Geometry: final body of the model. Coordinates: model frame, mm. Give positions to 0.01 mm unless a question says otherwise; leave off trailing zeros. Write each loop counter-clockwise with the first axis right and the second up, starting at its lowest first coordinate (ties: lowest second). Pieces come first, ordered by that corner, then holes.
```python
from build123d import *

# Parameters (mm, degrees)
F0_R     = 1.75
F1_DEPTH = 2.5


with BuildPart() as f1:
    # F0 (on Top) → F1 (new body)
    with BuildSketch(Plane.XY):
        with BuildLine():
            ThreePointArc((-38.5, -35.5), (-37.62132, -37.62132), (-35.5, -38.5))
            Line((-35.5, -38.5), (-2, -38.5))
            Line((-2, -38.5), (-2, -38.448017))
            ThreePointArc((-2, -38.448017), (-1.000338, -38.487002), (0, -38.5))
            ThreePointArc((0, -38.5), (1.000338, -38.487002), (2, -38.448017))
            Line((2, -38.448017), (2, -38.5))
            Line((2, -38.5), (35.5, -38.5))
            ThreePointArc((35.5, -38.5), (37.62132, -37.62132), (38.5, -35.5))
            Line((38.5, -35.5), (38.5, -2))
            Line((38.5, -2), (38.448017, -2))
            ThreePointArc((38.448017, -2), (38.487002, -1.000338), (38.5, 0))
            ThreePointArc((38.5, 0), (38.487002, 1.000338), (38.448017, 2))
            Line((38.448017, 2), (38.5, 2))
            Line((38.5, 2), (38.5, 35.5))
            ThreePointArc((38.5, 35.5), (37.62132, 37.62132), (35.5, 38.5))
            Line((35.5, 38.5), (2, 38.5))
            Line((2, 38.5), (2, 38.448017))
            ThreePointArc((2, 38.448017), (1.000338, 38.487002), (0, 38.5))
            ThreePointArc((0, 38.5), (-1.000338, 38.487002), (-2, 38.448017))
            Line((-2, 38.448017), (-2, 38.5))
            Line((-2, 38.5), (-35.5, 38.5))
            ThreePointArc((-35.5, 38.5), (-37.62132, 37.62132), (-38.5, 35.5))
            Line((-38.5, 35.5), (-38.5, 2))
            Line((-38.5, 2), (-38.448017, 2))
            ThreePointArc((-38.448017, 2), (-38.487002, 1.000338), (-38.5, 0))
            ThreePointArc((-38.5, 0), (-38.487002, -1.000338), (-38.448017, -2))
            Line((-38.448017, -2), (-38.5, -2))
            Line((-38.5, -2), (-38.5, -35.5))
        make_face()
        with Locations((-35, -35)):
            Circle(F0_R, mode=Mode.SUBTRACT)
        with BuildLine():
            Line((-16.039015, -35), (-31.045212, -35))
            ThreePointArc((-31.045212, -35), (-31.075605, -34.510637), (-31.166319, -34.028796))
            Line((-31.166319, -34.028796), (-25.754724, -28.617201))
            ThreePointArc((-25.754724, -28.617201), (-21.139162, -32.177412), (-16.039015, -35))
        make_face(mode=Mode.SUBTRACT)
        with BuildLine():
            ThreePointArc((-33.974785, -31.180408), (-34.482954, -31.079157), (-35, -31.045212))
            Line((-35, -31.045212), (-35, -16.039015))
            ThreePointArc((-35, -16.039015), (-32.164167, -21.159309), (-28.584922, -25.790545))
            Line((-28.584922, -25.790545), (-33.974785, -31.180408))
        make_face(mode=Mode.SUBTRACT)
        with BuildLine():
            Line((-2, -28.429738), (-2, -34.94281))
            ThreePointArc((-2, -34.94281), (-24.748737, -24.748737), (-34.94281, -2))
            Line((-34.94281, -2), (-28.429738, -2))
            ThreePointArc((-28.429738, -2), (-20.152543, -20.152543), (-2, -28.429738))
        make_face(mode=Mode.SUBTRACT)
        with BuildLine():
            Line((-2, -4.862478), (-2, -14.866069))
            ThreePointArc((-2, -14.866069), (-10.606602, -10.606602), (-14.866069, -2))
            Line((-14.866069, -2), (-4.794377, -2))
            Line((-4.794377, -2), (-8.49896, -8.49896))
            Line((-8.49896, -8.49896), (-2, -4.862478))
        make_face(mode=Mode.SUBTRACT)
        with BuildLine():
            ThreePointArc((-11.571705, -14.434183), (0.024219, -18.499984), (11.609459, -14.403835))
            Line((11.609459, -14.403835), (16.22518, -19.019557))
            ThreePointArc((16.22518, -19.019557), (0.024155, -24.999988), (-16.188397, -19.050874))
            Line((-16.188397, -19.050874), (-11.571705, -14.434183))
        make_face(mode=Mode.SUBTRACT)
        with BuildLine():
            Line((25.790545, -28.584922), (31.180408, -33.974785))
            ThreePointArc((31.180408, -33.974785), (31.079157, -34.482954), (31.045212, -35))
            Line((31.045212, -35), (16.039015, -35))
            ThreePointArc((16.039015, -35), (21.159309, -32.164167), (25.790545, -28.584922))
        make_face(mode=Mode.SUBTRACT)
        with Locations((35, -35)):
            Circle(F0_R, mode=Mode.SUBTRACT)
        with BuildLine():
            Line((35, -16.039015), (35, -31.045212))
            ThreePointArc((35, -31.045212), (34.510637, -31.075605), (34.028796, -31.166319))
            Line((34.028796, -31.166319), (28.617201, -25.754724))
            ThreePointArc((28.617201, -25.754724), (32.177412, -21.139162), (35, -16.039015))
        make_face(mode=Mode.SUBTRACT)
        with BuildLine():
            ThreePointArc((2, -28.429738), (20.152543, -20.152543), (28.429738, -2))
            Line((28.429738, -2), (34.94281, -2))
            ThreePointArc((34.94281, -2), (24.748737, -24.748737), (2, -34.94281))
            Line((2, -34.94281), (2, -28.429738))
        make_face(mode=Mode.SUBTRACT)
        with BuildLine():
            ThreePointArc((14.866069, -2), (10.606602, -10.606602), (2, -14.866069))
            Line((2, -14.866069), (2, -4.862478))
            Line((2, -4.862478), (8.49896, -8.49896))
            Line((8.49896, -8.49896), (4.794377, -2))
            Line((4.794377, -2), (14.866069, -2))
        make_face(mode=Mode.SUBTRACT)
        with BuildLine():
            ThreePointArc((-19.019557, -16.22518), (-25, 0), (-19.019557, 16.22518))
            Line((-19.019557, 16.22518), (-14.403835, 11.609459))
            ThreePointArc((-14.403835, 11.609459), (-18.5, 0), (-14.403835, -11.609459))
            Line((-14.403835, -11.609459), (-19.019557, -16.22518))
        make_face(mode=Mode.SUBTRACT)
        with BuildLine():
            ThreePointArc((-14.866069, 2), (-10.606602, 10.606602), (-2, 14.866069))
            Line((-2, 14.866069), (-2, 4.862478))
            Line((-2, 4.862478), (-8.49896, 8.49896))
            Line((-8.49896, 8.49896), (-4.794377, 2))
            Line((-4.794377, 2), (-14.866069, 2))
        make_face(mode=Mode.SUBTRACT)
        with BuildLine():
            ThreePointArc((-34.94281, 2), (-24.748737, 24.748737), (-2, 34.94281))
            Line((-2, 34.94281), (-2, 28.429738))
            ThreePointArc((-2, 28.429738), (-20.152543, 20.152543), (-28.429738, 2))
            Line((-28.429738, 2), (-34.94281, 2))
        make_face(mode=Mode.SUBTRACT)
        with BuildLine():
            Line((-33.974785, 31.180408), (-28.584922, 25.790545))
            ThreePointArc((-28.584922, 25.790545), (-32.164167, 21.159309), (-35, 16.039015))
            Line((-35, 16.039015), (-35, 31.045212))
            ThreePointArc((-35, 31.045212), (-34.482954, 31.079157), (-33.974785, 31.180408))
        make_face(mode=Mode.SUBTRACT)
        with Locations((-35, 35)):
            Circle(F0_R, mode=Mode.SUBTRACT)
        with BuildLine():
            ThreePointArc((-31.166319, 34.028796), (-31.075605, 34.510637), (-31.045212, 35))
            Line((-31.045212, 35), (-16.039015, 35))
            ThreePointArc((-16.039015, 35), (-21.139162, 32.177412), (-25.754724, 28.617201))
            Line((-25.754724, 28.617201), (-31.166319, 34.028796))
        make_face(mode=Mode.SUBTRACT)
        with BuildLine():
            ThreePointArc((2, 14.866069), (10.606602, 10.606602), (14.866069, 2))
            Line((14.866069, 2), (4.794377, 2))
            Line((4.794377, 2), (8.49896, 8.49896))
            Line((8.49896, 8.49896), (2, 4.862478))
            Line((2, 4.862478), (2, 14.866069))
        make_face(mode=Mode.SUBTRACT)
        with BuildLine():
            ThreePointArc((28.429738, 2), (20.152543, 20.152543), (2, 28.429738))
            Line((2, 28.429738), (2, 34.94281))
            ThreePointArc((2, 34.94281), (24.748737, 24.748737), (34.94281, 2))
            Line((34.94281, 2), (28.429738, 2))
        make_face(mode=Mode.SUBTRACT)
        with BuildLine():
            ThreePointArc((14.434183, -11.571705), (18.5, 0), (14.434183, 11.571705))
            Line((14.434183, 11.571705), (19.050874, 16.188397))
            ThreePointArc((19.050874, 16.188397), (25, 0), (19.050874, -16.188397))
            Line((19.050874, -16.188397), (14.434183, -11.571705))
        make_face(mode=Mode.SUBTRACT)
        with BuildLine():
            ThreePointArc((11.609459, 14.403835), (0.024219, 18.499984), (-11.571705, 14.434183))
            Line((-11.571705, 14.434183), (-16.188397, 19.050874))
            ThreePointArc((-16.188397, 19.050874), (0.024155, 24.999988), (16.22518, 19.019557))
            Line((16.22518, 19.019557), (11.609459, 14.403835))
        make_face(mode=Mode.SUBTRACT)
        with BuildLine():
            ThreePointArc((34.028796, 31.166319), (34.510637, 31.075605), (35, 31.045212))
            Line((35, 31.045212), (35, 16.039015))
            ThreePointArc((35, 16.039015), (32.177412, 21.139162), (28.617201, 25.754724))
            Line((28.617201, 25.754724), (34.028796, 31.166319))
        make_face(mode=Mode.SUBTRACT)
        with BuildLine():
            ThreePointArc((25.790545, 28.584922), (21.159309, 32.164167), (16.039015, 35))
            Line((16.039015, 35), (31.045212, 35))
            ThreePointArc((31.045212, 35), (31.079157, 34.482954), (31.180408, 33.974785))
            Line((31.180408, 33.974785), (25.790545, 28.584922))
        make_face(mode=Mode.SUBTRACT)
        with Locations((35, 35)):
            Circle(F0_R, mode=Mode.SUBTRACT)
    extrude(amount=F1_DEPTH)


solid = f1.part
```
Item 1: Section A-A, the plane y = -3. Return the cut outline in (x, z).
Found:
outline: (-38.5, 0) - (-34.87, 0) - (-34.87, 2.5) - (-38.5, 2.5) - close; (-28.34, 0) - (-24.82, 0) - (-24.82, 2.5) - (-28.34, 2.5) - close; (-18.26, 0) - (-14.7, 0) - (-14.7, 2.5) - (-18.26, 2.5) - close; (-5.36, 0) - (5.36, 0) - (5.36, 2.5) - (-5.36, 2.5) - close; (14.7, 0) - (18.26, 0) - (18.26, 2.5) - (14.7, 2.5) - close; (24.82, 0) - (28.34, 0) - (28.34, 2.5) - (24.82, 2.5) - close; (34.87, 0) - (38.5, 0) - (38.5, 2.5) - (34.87, 2.5) - close
Item 2: Pull-direction query (Y, two-part tool) for faces 1 (the face through (-19, 38.5, 1)), 2 (the face through (-1, 1, 2.5)), 3 (the face through (32, 2, 1)); classes: +Y half, -Y half, draft (parallel to the pull), parting line (faces both ways), or undercut.
Found:
face 1: +Y half
face 2: draft
face 3: undercut
Item 3: Section D-D, the plane z = 0.45. State how many separate pieces and enclosed holes the cut face has, plus the area to 3 significant figures.
Found:
separate pieces: 1
enclosed holes: 24
area: 3,120 mm2
Item 4: Section B-B, the plane x = -22.5. Return the cut outline in (y, z).
Found:
outline: (-38.5, 0) - (-35, 0) - (-35, 2.5) - (-38.5, 2.5) - close; (-31.24, 0) - (-26.81, 0) - (-26.81, 2.5) - (-31.24, 2.5) - close; (-17.49, 0) - (-10.9, 0) - (-10.9, 2.5) - (-17.49, 2.5) - close; (10.9, 0) - (17.49, 0) - (17.49, 2.5) - (10.9, 2.5) - close; (26.81, 0) - (31.24, 0) - (31.24, 2.5) - (26.81, 2.5) - close; (35, 0) - (38.5, 0) - (38.5, 2.5) - (35, 2.5) - close
Item 5: Section C-C, the plane y = -24. Return the cut outline in (x, z), plus the area to 3 significant figures.
Found:
outline: (-38.5, 0) - (-35, 0) - (-35, 2.5) - (-38.5, 2.5) - close; (-30.1, 0) - (-25.48, 0) - (-25.48, 2.5) - (-30.1, 2.5) - close; (-15.37, 0) - (-7, 0) - (-7, 2.5) - (-15.37, 2.5) - close; (7, 0) - (15.37, 0) - (15.37, 2.5) - (7, 2.5) - close; (25.48, 0) - (30.1, 0) - (30.1, 2.5) - (25.48, 2.5) - close; (35, 0) - (38.5, 0) - (38.5, 2.5) - (35, 2.5) - close
area: 82.5 mm2
Item 6: Line query: L1, parallel to X at y = -23, z = 1.6; L2, parallel to X at y = 20, z = 0.6. Output: solid intervals per line, ascending.
Found:
L1: x = -38.5 to -35, -30.87 to -26.38, -16.83 to -9.8, 9.8 to 16.83, 26.38 to 30.87, 35 to 38.5
L2: x = -38.5 to -35, -32.9 to -28.72, -20.3 to -15, 15 to 20.3, 28.72 to 32.9, 35 to 38.5
